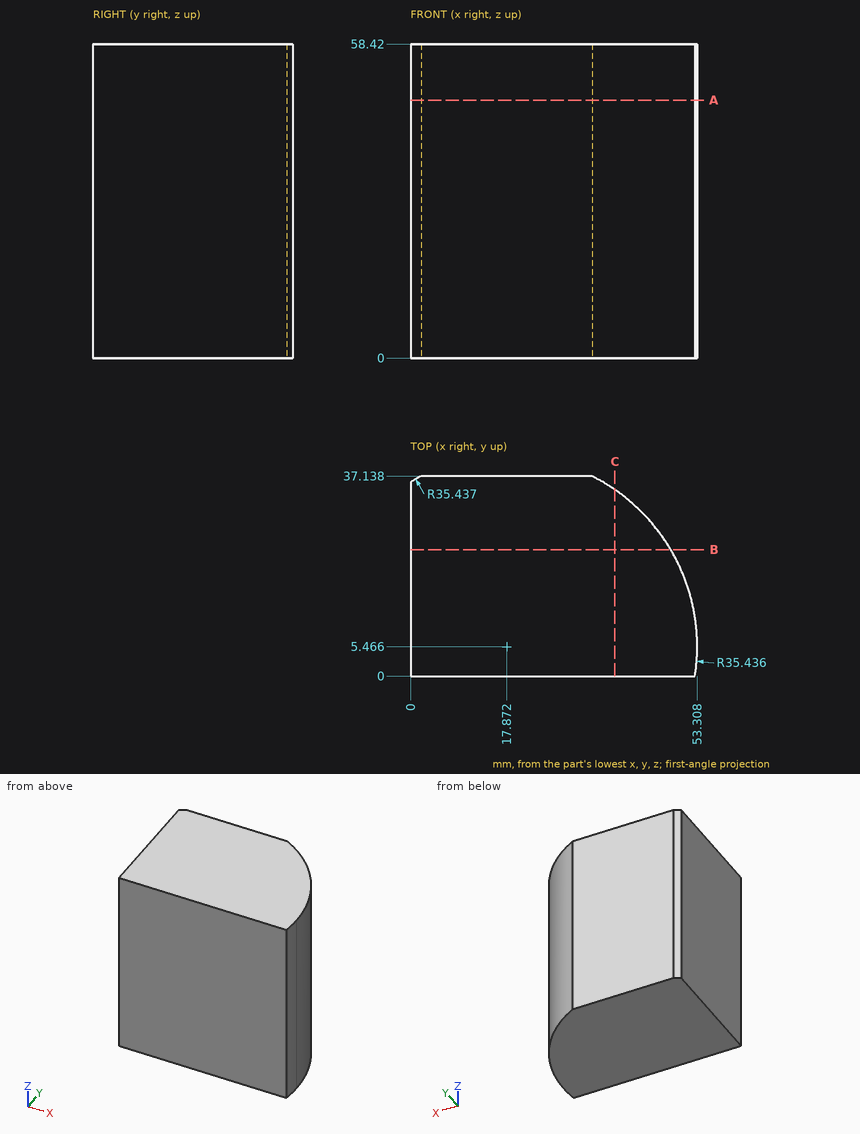
Here's the drawing with two shaded views (mm, measured from the low corner). I have some questions. Coordinates: 2 decimals unless noted, no trailing zeros. Order: outer loops, then holes, each group sorted by start corner. A loop starts at its lowest first (then second) coordinate and runs counter-clockwise, first axis right, second up. Notation, with made-up numbers: (-6.75, 73) - (38.25, 73) arc R16 cw to (38.25, 78) - close; hole circle Ø3 at (62.5, -1). An arc over 180 degrees is marked (long way). Use CSV: the item, a comma, the result in double quotes. Start each with the question number.
1. I'm going to push flat-ended pins straight in: pin 1 (2 mm diameter, centred on y = 29.5, z = 21.5, fed in from +X); pin 2 (1 mm diameter, centred on x = 41.5, z = 17.5, fed in from +Y) (1 decimal). Where does each tip first touch, or does it pass through?
2. Suppose I cut it at C-C on x = 38. List the corners of the cut face in (y, z) for me.
3. Please list where these lines run through material, in increasing order: line 1 (X direction, y = 6, z = 20) (1 decimal); line 2 (Y direction, x = 45, z = 24) (1 decimal); line 3 (X direction, y = 20, z = 14.5). Write a range as from..to.
4. Suppose I cut it at B-B on y = 23.5. List the corners of the cut face in (x, z) for me, then the cut area to 3 significant figures.
5. Suppose I cut it at A-A on z = 48. List the corners of the cut face in (x, y) for me (1 decimal), then the cut area to 3 significant figures.
Output:
1,pin 1,"stops at x = 44.8"
1,pin 2,"stops at y = 32.3"
2,outline,"(0, 0) - (34.63, 0) - (34.63, 58.42) - (0, 58.42) - close"
3,line 1,"x = 0..53.3"
3,line 2,"y = 0..28.3"
3,line 3,"x = 0..50.19"
4,outline,"(0, 0) - (48.38, 0) - (48.38, 58.42) - (0, 58.42) - close"
4,area,"2,830 mm2"
5,outline,"(0, 0) - (52.9, 0) arc R35.4 ccw to (53.3, 5.5) arc R35.4 ccw to (33.8, 37.1) - (2, 37.1) arc R35.4 ccw to (0, 36.1) - close"
5,area,"1,800 mm2"
